```python
from build123d import *

# Parameters (mm, degrees)
F1_DEPTH  = 10
F2_W      = 40.3112887415
F2_H      = 2
F3_DEPTH  = 12
F6_DEPTH  = 10
F7_W      = 12
F7_H      = 10
F8_DEPTH  = 40
F9_W      = 59.6965367126
F9_H      = 7.6070292853
F10_DEPTH = 25


# Not quite as in the source:
# - a feature of the source that left no trace in its solid (it failed there, or was rolled back) is left out


with BuildPart() as f1:
    # F0 (on Front) → F1 (new body)
    with BuildSketch(Plane.XZ):
        with BuildLine():
            ThreePointArc((-6, 21.6852484422), (-13.6244265934, -17.9060045795), (22.5, 0))
            ThreePointArc((22.5, 0), (17.9060045795, 13.6244265934), (6, 21.6852484422))
            ThreePointArc((6, 21.6852484422), (3.0275328281, 22.2953816961), (0, 22.5))
            ThreePointArc((0, 22.5), (-3.0275328281, 22.2953816961), (-6, 21.6852484422))
        make_face()
    extrude(amount=F1_DEPTH)

    # F2 (on face) → F3 (join)
    with BuildSketch(Plane.XZ.offset(10)):
        with Locations((0, 9)):
            Rectangle(F2_W, F2_H)
        with Locations((0, -9)):
            Rectangle(F2_W, F2_H)
        with BuildLine():
            Line((20.1556443707, 10), (20.1556443707, 8))
            Line((20.1556443707, 8), (21.0297408448, 8))
            ThreePointArc((21.0297408448, 8), (20.6169587679, 9.0106054825), (20.1556443707, 10))
        make_face()
        with BuildLine():
            ThreePointArc((-20.1556443707, 10), (-20.6169587679, 9.0106054825), (-21.0297408448, 8))
            Line((-21.0297408448, 8), (-20.1556443707, 8))
            Line((-20.1556443707, 8), (-20.1556443707, 10))
        make_face()
        with BuildLine():
            Line((-20.1556443707, -8), (-21.0297408448, -8))
            ThreePointArc((-21.0297408448, -8), (-20.6169587679, -9.0106054825), (-20.1556443707, -10))
            Line((-20.1556443707, -10), (-20.1556443707, -8))
        make_face()
        with BuildLine():
            Line((21.0297408448, -8), (20.1556443707, -8))
            Line((20.1556443707, -8), (20.1556443707, -10))
            ThreePointArc((20.1556443707, -10), (20.6169587679, -9.0106054825), (21.0297408448, -8))
        make_face()
    extrude(amount=F3_DEPTH)

    # F0 (on Front) → F6 (join)
    with BuildSketch(Plane.XZ):
        with BuildLine():
            ThreePointArc((-6, 21.6852484422), (-13.6244265934, -17.9060045795), (22.5, 0))
            ThreePointArc((22.5, 0), (17.9060045795, 13.6244265934), (6, 21.6852484422))
            ThreePointArc((6, 21.6852484422), (3.0275328281, 22.2953816961), (0, 22.5))
            ThreePointArc((0, 22.5), (-3.0275328281, 22.2953816961), (-6, 21.6852484422))
        make_face()
        with BuildLine():
            ThreePointArc((0, 22.5), (3.0275328281, 22.2953816961), (6, 21.6852484422))
            Line((6, 21.6852484422), (6, 22.5))
            Line((6, 22.5), (0, 22.5))
        make_face()
        with BuildLine():
            Line((-6, 22.5), (-6, 21.6852484422))
            ThreePointArc((-6, 21.6852484422), (-3.0275328281, 22.2953816961), (0, 22.5))
            Line((0, 22.5), (-6, 22.5))
        make_face()
    extrude(amount=F6_DEPTH)

    # F7 (on face) → F8 (join)
    with BuildSketch(Plane.XY.offset(22.5)):
        with Locations((0, -5)):
            Rectangle(F7_W, F7_H)
    extrude(amount=F8_DEPTH)

    # F9 (on face) → F10 (cut)
    with BuildSketch(Plane.XY.offset(6)):
        with Locations((-0.8811633027, 3.8035146426)):
            Rectangle(F9_W, F9_H)
    extrude(amount=-F10_DEPTH, mode=Mode.SUBTRACT)


solid = f1.part
```
For this review, take the finished solid that the model builds, in its own axes (mm). A direction names the side the tool comes from. Give positions to 0.01 mm unless a question says otherwise; leave off trailing zeros. Write each loop counter-clockwise with the first axis right and the second up, starting at its lowest first coordinate (ties: lowest second). Pieces come first, ordered by that corner, then holes. Notation, with made-up numbers: M 73.25,70 L 106.25,70 A28 cw 106.25,100 Z; hole C 19,15 d7. An arc over 180 degrees is marked long. Answer as a JSON object with one key per item and string values. Group by question number.
Item 1: Consider section C-C on z = 44. Write out the cut boundary in (x, y).
Item 2: Tool access review of faces 1 (the flat face through (6, -5, 42)), 2 (the flat face through (0, -10, 0)), 3 (the flat face through (0, -10, -15)), 4 (the flat face through (0, -16, 10)), 5 (the flat face through (-6, -5, 42)): name each direction out of +Z, -Z, +X, -X, +Y, -Y from which nothing blocks a thin tool from reaching the whole face with its end or side.
Item 3: Draft analysis for pull direction Z (two halves, no side actions). For faces 6 (the flat face through (0, -22, -9)), 7 (the flat face through (0, -16, -8)), 8 (the flat face through (0, -16, 8)), 9 (the flat face through (0, -5, 62.5)), state which applies: +Z half, -Z half, draft (parallel to the pull), parting line (faces both ways), or undercut.
Item 4: Consider section A-A on y = -19.5. Write out the cut boundary in (x, z), plus the area to 3 significant figures.
Item 5: Consider section B-B on x = 0. Write out the cut boundary in (y, z), plus the area to 3 significant figures.
Item 6: For pin 1 Ø6 at (x, y) = (7, -16.5) entering from -Z; pin 2 Ø5 at (x, z) = (-6.5, 2.5) entering from -Y; pin 3 Ø9.5 at (x, y) = (-4, -18.5) entering from +Z; pin 4 Ø3 at (y, z) = (-13, 40.5) entering from -X, all flat-tipped, find the tip position at first contact; note any pin that passes through.
Item 7: For probe 1 along Z at (x, y) = (-13.5, -14.5); probe 2 along Y at (x, z) = (2.5, 53); probe 3 along X at (y, z) = (-7.5, 46.5), list the stretches that pass through material, from the lowest coordinate up. Write a range as [from, to].
Item 8: Consider section D-D on y = -3.75. Write out the cut boundary in (x, z), plus the area to 3 significant figures.
Check result:
{
 "1": {"outline": "M -6,-10 L 6,-10 L 6,0 L -6,0 Z"},
 "2": {"face 1": "+Z, +X, +Y, -Y", "face 2": "+X, -X, -Y", "face 3": "-Z, +X, -X, -Y", "face 4": "+Z, +X, -X, -Y", "face 5": "+Z, -X, +Y, -Y"},
 "3": {"face 6": "draft", "face 7": "undercut", "face 8": "undercut", "face 9": "+Z half"},
 "4": {"outline": "M -21.03,-8 A22.5 ccw -20.16,-10 L 20.16,-10 A22.5 ccw 21.03,-8 Z; M -21.03,8 L 21.03,8 A22.5 ccw 20.16,10 L -20.16,10 A22.5 ccw Z", "area": "165 mm^2"},
 "5": {"outline": "M -22,-10 L -10,-10 L -10,-22.5 L 0,-22.5 L 0,62.5 L -10,62.5 L -10,10 L -22,10 L -22,8 L -10,8 L -10,-8 L -22,-8 Z", "area": "898 mm^2"},
 "6": {"pin 1": "stops at z = -10", "pin 2": "stops at y = -10", "pin 3": "stops at z = 10", "pin 4": "passes through"},
 "7": {"probe 1": "z = [-10, -8], [8, 10]", "probe 2": "y = [-10, 0]", "probe 3": "x = [-6, 6]"},
 "8": {"outline": "M -6,21.69 A22.5 ccw long 6,21.69 L 6,62.5 L -6,62.5 Z", "area": "2,070 mm^2"}
}
